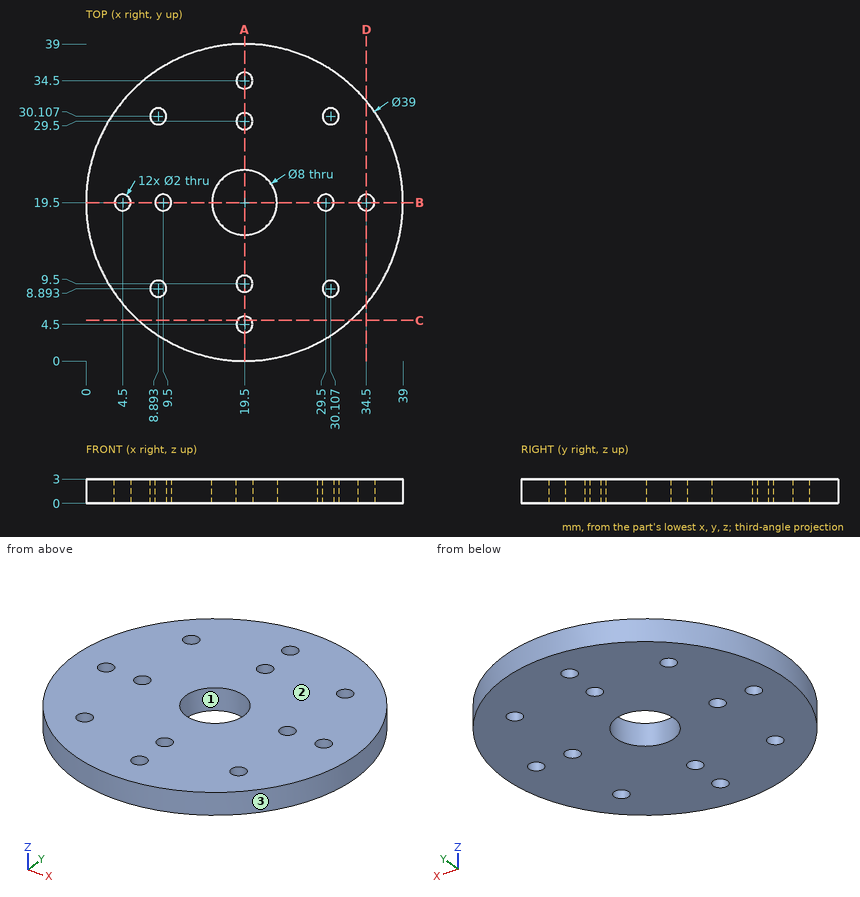
For this review, use the dimensioned drawing (mm, ordinates from the lowest corner) and the shaded views. Coordinates: 2 decimals unless noted, no trailing zeros. Loops run counter-clockwise (first coordinate to the right, second up) from the corner with the lowest first, then second, coordinate; pieces in that order, holes last. Notation, with made-up numbers: (66.25, 59) -> (103.25, 59) arc R11 cw to (103.25, 77) -> close; hole circle Ø9 at (57, 63.25). An arc over 180 degrees is marked (long way). Write each question's results on one line, items separated by ' | '.
Q1. Mouldability with a two-part tool opening along Y and no side actions: class the marked faces 1, 2 and 3 as +Y half, -Y half, draft (parallel to the pull), parting line (faces both ways), or undercut.
Taken from the geometry:
face 1: undercut | face 2: draft | face 3: parting line
Q2. For pin 1 Ø1.5 at (y, z) = (6.5, 1) entering from +X; pin 2 Ø1.2 at (x, y) = (29.5, 19.5) entering from -Z; pin 3 Ø1 at (x, z) = (32.5, 1) entering from +Y, all flat-tipped, find the tip position at first contact; note any pin that passes through.
Taken from the geometry:
pin 1: x = 34.67 | pin 2: through | pin 3: y = 34.47
Q3. Add section A-A, the plane x = 19.5. State the section outline as (y, z) points.
Taken from the geometry:
outline: (0, 0) -> (3.5, 0) -> (3.5, 3) -> (0, 3) -> close; (5.5, 0) -> (8.5, 0) -> (8.5, 3) -> (5.5, 3) -> close; (10.5, 0) -> (15.5, 0) -> (15.5, 3) -> (10.5, 3) -> close; (23.5, 0) -> (28.5, 0) -> (28.5, 3) -> (23.5, 3) -> close; (30.5, 0) -> (33.5, 0) -> (33.5, 3) -> (30.5, 3) -> close; (35.5, 0) -> (39, 0) -> (39, 3) -> (35.5, 3) -> close
Q4. Add section D-D, the plane x = 34.5. State the section outline as (y, z) points.
Taken from the geometry:
outline: (7.04, 0) -> (18.5, 0) -> (18.5, 3) -> (7.04, 3) -> close; (20.5, 0) -> (31.96, 0) -> (31.96, 3) -> (20.5, 3) -> close
Q5. Add section C-C, the plane y = 5. State the section outline as (x, z) points.
Taken from the geometry:
outline: (6.46, 0) -> (18.63, 0) -> (18.63, 3) -> (6.46, 3) -> close; (20.37, 0) -> (32.54, 0) -> (32.54, 3) -> (20.37, 3) -> close
Q6. To check wall thickness, follow line 1 along Y through (x, z) = (19.5, 1.6); line 2 along Y through (x, z) = (29.5, 1.9); line 3 along Y through (x, z) = (34, 0.8) (1 decimal). State the ranges of each line that lie inside material, in increasing order. Write a range as [from, to].
Taken from the geometry:
line 1: [0, 3.5], [5.5, 8.5], [10.5, 15.5], [23.5, 28.5], [30.5, 33.5], [35.5, 39] | line 2: [2.76, 8.1], [9.69, 18.5], [20.5, 29.31], [30.9, 36.24] | line 3: [6.5, 18.6], [20.4, 32.5]
